Input: part model. Units: mm. Frame: model coordinates. Face numbers are marked on the shaded views. Give positions to 0.01 mm unless a question says otherwise; leave off trailing zeros. Order: outer loops, then holes, each group sorted by start corner. A loop starts at its lowest first (then second) coordinate and runs counter-clockwise, first axis right, second up.
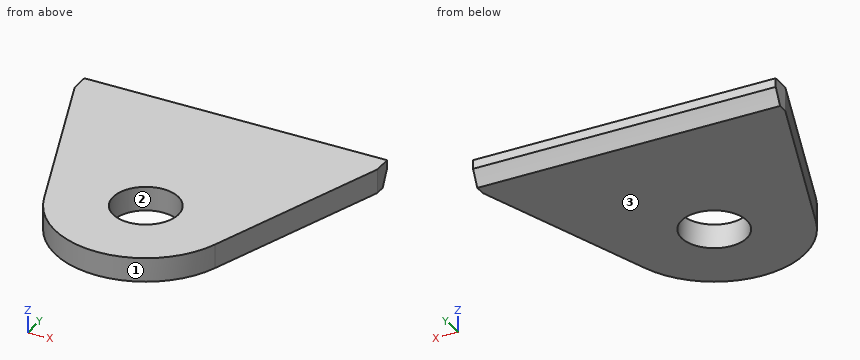
```python
from build123d import *

# Parameters (mm, degrees)
SKETCH_1_R                 = 5.4
EXTRUDE_1_DEPTH            = 4
CUT_EXTRUDE_534_DEPTH      = 38.749172176
CUT_EXTRUDE_534_DEPTH_BACK = 38.749172176
SKETCH_514_R               = 66.5


with BuildPart() as part:
    # Эскиз1 → Бобышка-Вытянуть1 (new body)
    with BuildSketch(Plane.XY):
        with BuildLine():
            Line((-25, 28), (25, 28))
            Line((25, 28), (25, 25))
            Line((25, 25), (14.104686356, -5.104686356))
            ThreePointArc((14.104686356, -5.104686356), (0, -15), (-14.104686356, -5.104686356))
            Line((-14.104686356, -5.104686356), (-25, 25))
            Line((-25, 25), (-25, 28))
        make_face()
        Circle(SKETCH_1_R, mode=Mode.SUBTRACT)
    extrude(amount=EXTRUDE_1_DEPTH)

    # Sketch 514 → Cut-Extrude 534 (cut, two sides: drawn at the far end of the back side and taken through both)
    with BuildSketch(Plane(origin=(0, 0, 0), x_dir=(0, 0, -1), z_dir=(1, 0, 0)).offset(-CUT_EXTRUDE_534_DEPTH_BACK)):
        with Locations((30, 86)):
            Circle(SKETCH_514_R)
    extrude(amount=CUT_EXTRUDE_534_DEPTH + CUT_EXTRUDE_534_DEPTH_BACK, mode=Mode.SUBTRACT)


solid = part.part
```
1) Line query: probe 1 along Y at (x, z) = (0, 2.9); probe 2 along Y at (x, z) = (-4.5, 2.8); probe 3 along X at (y, z) = (-3, 1.75). Output: solid intervals per line, ascending.
2) First-contact query: P1, Ø12, axis at x = 17, y = 10.5, coming from the -Z side; P2, Ø2, axis at y = -3.5, z = 0.5, coming from the -X side. Flat tips, straight axial feed; report the tip coordinate or a pass-through.
3) Cut plane B-B (y = 0). Return the cut outline in (x, z).
4) Cut plane D-D (x = -13). Return the cut outline in (y, z).
5) Cut plane A-A (x = 0). Return the cut outline in (y, z), then the cut area to 3 significant figures.
6) Cut plane C-C (z = 1.3). Return the cut outline in (x, y), then the cut area to 3 significant figures.
7) Pull-direction query (Y, two-part tool) for the marked faces 1, 2 and 3; classes: pulls with the +Y half, pulls with the -Y half, needs draft (parallel to the pull), parting line crosses it, or undercut.
Geometry says:
1. probe 1: y = -15 to -5.4, 5.4 to 28
1. probe 2: y = -14.31 to -2.98, 2.98 to 28
1. probe 3: x = -14.87 to -4.49, 4.49 to 14.87
2. P1: stops at z = 0
2. P2: stops at x = -15.05
3. outline: (-15.95, 0) - (-5.4, 0) - (-5.4, 4) - (-15.95, 4) - close; (5.4, 0) - (15.95, 0) - (15.95, 4) - (5.4, 4) - close
4. outline: (-7.48, 0) - (26.65, 0) arc R66.5 cw to (28, 2.53) - (28, 4) - (-7.48, 4) - close
5. outline: (-15, 0) - (-5.4, 0) - (-5.4, 4) - (-15, 4) - close; (5.4, 0) - (26.65, 0) arc R66.5 cw to (28, 2.53) - (28, 4) - (5.4, 4) - close
5. area: 127 mm2
6. outline: (-25, 25) - (-14.1, -5.1) arc R15 ccw to (14.1, -5.1) - (25, 25) - (25, 27.33) - (-25, 27.33) - close; hole circle Ø10.8 at (0, 0)
6. area: 1,410 mm2
7. face 1: pulls with the -Y half
7. face 2: undercut
7. face 3: needs draft
